Design review of the part built by this model. Coordinates are the model's own, in mm. A direction names the side the tool comes from. Give positions to 0.01 mm unless a question says otherwise; leave off trailing zeros. Write each loop counter-clockwise with the first axis right and the second up, starting at its lowest first coordinate (ties: lowest second). Pieces come first, ordered by that corner, then holes.
```python
from build123d import *

# Parameters (mm, degrees)
SKETCH1_W           = 38.1
SKETCH1_H           = 76.2
BOSS_EXTRUDE1_DEPTH = 7.9375
SKETCH2_R           = 3.96875
CUT_EXTRUDE1_DEPTH  = 44.330317403
SKETCH4_R           = 9.525
CUT_EXTRUDE2_DEPTH  = 4.7625
SKETCH5_R           = 4.7625
BOSS_EXTRUDE2_DEPTH = 9.4488
SKETCH6_R           = 3.175
BOSS_EXTRUDE3_DEPTH = 6.604


with BuildPart() as part:
    # Sketch1 → Boss-Extrude1 (new body)
    with BuildSketch(Plane.XY):
        Rectangle(SKETCH1_W, SKETCH1_H)
    extrude(amount=BOSS_EXTRUDE1_DEPTH)

    # Sketch2 → Cut-Extrude1 (cut, through all)
    with BuildSketch(Plane.XY.offset(7.9375)):
        Circle(SKETCH2_R)
    extrude(amount=-CUT_EXTRUDE1_DEPTH, mode=Mode.SUBTRACT)

    # Sketch4 → Cut-Extrude2 (cut)
    with BuildSketch(Plane.XY.offset(7.9375)):
        Circle(SKETCH4_R)
    extrude(amount=-CUT_EXTRUDE2_DEPTH, mode=Mode.SUBTRACT)

    # Sketch5 → Boss-Extrude2 (add)
    with BuildSketch(Plane.XY.offset(7.9375)):
        with Locations(Location((0, 25.4, 0), (0, 0, 180))):
            Circle(SKETCH5_R)
    boss_extrude2 = extrude(amount=BOSS_EXTRUDE2_DEPTH)

    # Sketch6 → Boss-Extrude3 (add)
    with BuildSketch(Plane.XY.offset(17.3863)):
        with Locations(Location((0, 25.4, 0), (0, 0, 180))):
            Circle(SKETCH6_R)
    boss_extrude3 = extrude(amount=BOSS_EXTRUDE3_DEPTH)

    # Mirror1: Boss-Extrude2, Boss-Extrude3 across plane
    add(boss_extrude2.mirror(Plane.ZX))
    add(boss_extrude3.mirror(Plane.ZX))


solid = part.part
```
(1) Consider section C-C, the plane z = 13. Give the boundary of the cut face in (x, y) (1 decimal), then the cut area to 3 significant figures.
Resolved:
outline: circle Ø9.5 at (0, -25.4); circle Ø9.5 at (0, 25.4)
area: 143 mm2
(2) Tool access review of faces 5 (the face through (0, 38.1, 4)), 6 (the face through (0.41, 22.25, 20.64)): name each direction out of +Z, -Z, +X, -X, +Y, -Y from which nothing blocks a thin tool from reaching the whole face with its end or side.
Resolved:
face 5: +Z, -Z, +X, -X, +Y
face 6: +Z
(3) Mouldability with a two-part tool opening along X and no side actions: class faces 1 (the face through (-0.86, -3.874, 1.61)), 2 (the face through (19.05, -1, 4)), 3 (the face through (-1, 29, 17.386)), 4 (the face through (-7.559, -5.796, 5.59)) as pulls with the +X half, pulls with the -X half, needs draft (parallel to the pull), parting line crosses it, or undercut.
Resolved:
face 1: undercut
face 2: pulls with the +X half
face 3: needs draft
face 4: undercut
(4) Consider section B-B, the plane x = 0. Give the boundary of the cut face in (y, z) (1 decimal), then the cut area to 3 significant figures.
Resolved:
outline: (-38.1, 0) - (-4, 0) - (-4, 3.2) - (-9.5, 3.2) - (-9.5, 7.9) - (-20.6, 7.9) - (-20.6, 17.4) - (-22.2, 17.4) - (-22.2, 24) - (-28.6, 24) - (-28.6, 17.4) - (-30.2, 17.4) - (-30.2, 7.9) - (-38.1, 7.9) - close; (4, 0) - (38.1, 0) - (38.1, 7.9) - (30.2, 7.9) - (30.2, 17.4) - (28.6, 17.4) - (28.6, 24) - (22.2, 24) - (22.2, 17.4) - (20.6, 17.4) - (20.6, 7.9) - (9.5, 7.9) - (9.5, 3.2) - (4, 3.2) - close
area: 753 mm2
(5) Clearance check with flat-ended pins moving along their axes: P1, Ø10.5, axis at x = 0, y = 0, coming from the +Z side (3 decimals); P2, Ø15, axis at x = -4.5, y = -3, coming from the +Z side; P3, Ø10, axis at y = 16, z = 14, coming from the -X side; P4, Ø1.5, axis at x = 4.5, z = 19, coming from the +Y side. State where each tip first meets the part, or that it passes through.
Resolved:
P1: stops at z = 3.175
P2: stops at z = 7.94
P3: stops at x = -1.82
P4: passes through
(6) To check wall thickness, follow L1, parallel to Y at x = 0, z = 0.6; L2, parallel to Y at x = 0, z = 6.7 (3 decimals); L3, parallel to Z at x = -2, y = 29.5. State the ranges of each line that lie inside material, in increasing order.
Resolved:
L1: y = -38.1 to -3.97, 3.97 to 38.1
L2: y = -38.1 to -9.525, 9.525 to 38.1
L3: z = 0 to 17.39
